For this review, take the finished solid that the model builds, in its own axes (mm). A direction names the side the tool comes from. Give positions to 0.01 mm unless a question says otherwise; leave off trailing zeros. Write each loop counter-clockwise with the first axis right and the second up, starting at its lowest first coordinate (ties: lowest second). Pieces come first, ordered by that corner, then holes. Notation, with made-up numbers: M -37,69 L -10,69 A29 ccw -10,96 Z; hole C 33.25,43 d7. An arc over 180 degrees is marked long. Write item = value, one per line.
Solid Edge part; units mm, degrees
sketch "Sketch1" plane through (0, 0, 0) normal (0, 0, 1) x (1, 0, 0)
  circle A0 centre (0, 0) radius 21.3
extrude "Protrusion1" add sketch "Sketch1" along normal blind 3
sketch "Sketch2" plane through (0, 0, 3) normal (0, 0, 1) x (1, 0, 0)
  circle A0 centre (0, 0) radius 23.3
extrude "ExtrudedProtrusion_2" add sketch "Sketch2" along normal blind 2
sketch "Sketch3" plane through (0, 0, 0) normal (0, 0, -1) x (1, 0, 0)
  circle A0 centre (0, 0) radius 19.3
extrude "ExtrudedCutout_1" cut sketch "Sketch3" against normal blind 3
sketch "Sketch4" plane through (0, 0, 5) normal (0, 0, 1) x (-1, 0, 0)
  circle A0 centre (0, 0) radius 1
extrude "ExtrudedCutout_2" cut sketch "Sketch4" against normal blind 2
1. The part is to be moulded in two halves that separate along X. For faces 3 (the face through (18.409, -5.797, 1.479)), 4 (the face through (0, 1, 4)), 5 (the face through (20.316, -6.398, 1.479)), 6 (the face through (5, 0, 5)), say which applies: +X half, -X half, draft (parallel to the pull), parting line (faces both ways), or undercut.
Responses:
face_3 = undercut
face_4 = undercut
face_5 = parting line
face_6 = draft
2. For line 1 along Y through (x, z) = (0, 3.65); line 2 along Y through (x, z) = (0, 1.3); line 3 along X through (y, z) = (-0.5, 2.5), list the stretches that pass through material, from the lowest coordinate up. Write a range as from..to.
Responses:
line_1 = -23.3..-1, 1..23.3
line_2 = -21.3..-19.3, 19.3..21.3
line_3 = -21.29..-19.29, 19.29..21.29
3. We need section A-A, the plane x = 0. Write out the cut boundary in (y, z).
Responses:
outline = M -23.3,3 L -21.3,3 L -21.3,0 L -19.3,0 L -19.3,3 L -1,3 L -1,5 L -23.3,5 Z; M 1,3 L 19.3,3 L 19.3,0 L 21.3,0 L 21.3,3 L 23.3,3 L 23.3,5 L 1,5 Z
4. Insertion check: P1, Ø1.5, axis at y = 11.5, z = 4, coming from the -X side; P2, Ø3, axis at x = -15, z = 1, coming from the -Y side; P3, Ø11.5, axis at x = -8.5, y = 1.5, coming from the -Z side. Each pin has a flat end and moves straight along its axis. Give the tip position at first contact, or say it passes through.
Responses:
P1 = -20.67
P2 = -16.48
P3 = 3
5. We need section D-D, the plane x = 13. Write out the cut boundary in (y, z) (3 decimals).
Responses:
outline = M -19.336,3 L -16.873,3 L -16.873,0 L -14.265,0 L -14.265,3 L 14.265,3 L 14.265,0 L 16.873,0 L 16.873,3 L 19.336,3 L 19.336,5 L -19.336,5 Z
6. Machinability: for faces 1 (the face through (-4, 0, 3)), 2 (the face through (-5.051, 22.746, 3.986)), which of the approach directions +Z, -Z, +X, -X, +Y, -Y give a long, thin tool a straight path to every point of the face, cutting with its end or side? Answer none if there is none.
Responses:
face_1 = -Z
face_2 = +Z, -Z
7. We need section C-C, the plane z = 1.5. Write out the cut boundary in (x, y).
Responses:
outline = C 0,0 d42.6; hole C 0,0 d38.6
